```python
from build123d import *

# Parameters (mm, degrees)
F1_DEPTH = 7
F3_D     = 10


with BuildPart() as f1:
    # F0 (on Front) → F1 (new body)
    with BuildSketch(Plane.XZ):
        Polygon((7.5, -4.330127), (7.5, 4.330127), (0, 8.660254), (-7.5, 4.330127), (-7.5, -4.330127), (0, -8.660254), align=None)
    extrude(amount=F1_DEPTH)

    # F3 (through all)
    with Locations(Plane.XZ.offset(7)):
        with Locations((0, 0)):
            Hole(F3_D / 2)


solid = f1.part
```
The model under review builds one solid part; all positions refer to its coordinate system, in mm. Round coordinates to 2 decimals unless told otherwise and drop trailing zeros. Order: outer loops, then holes, each group sorted by start corner. A loop starts at its lowest first (then second) coordinate and runs counter-clockwise, first axis right, second up. Notation, with made-up numbers: (-28, 25.25) -> (23, 25.25) arc R15 ccw to (23, 50.25) -> close; hole circle Ø10 at (83.25, 73.5). An arc over 180 degrees is marked (long way). One line per item, written item: value. Start each with the question number.
Q1. Take a section at A-A (z = 0). Write out the cut boundary in (x, y), and give its area (3 significant figures).
Q2. Take a section at B-B (y = -3). Write out the cut boundary in (x, z).
Q3. Mouldability with a two-part tool opening along X and no side actions: class faces 1 (the face through (1.08, -3.45, -4.88)), 2 (the face through (-5, 0, -2)), 3 (the face through (-3.802, -3.451, -6.465)), 4 (the face through (7.5, -3, 0)) as released by +X, released by -X, zero draft, split by the parting line, or undercut.
Q4. Wall thickness on line 1 (Z direction, x = -4.25, y = -5.5); line 2 (X direction, y = -5, z = -4.5); line 3 (X direction, y = -0.75, z = -1.25): over which ranges is each line inside the solid? List them lowest first.
Q5. Clearance check with a flat-ended pin moving along its axis: pin 1 Ø1 at (x, y) = (2, -4.5) entering from +Z. State where the tip first meets the part, or that it passes through.
Q6. Take a section at D-D (z = 7.75). Write out the cut boundary in (x, y), and give its area (3 significant figures).
Q7. Take a section at C-C (x = -1.25). Write out the cut boundary in (y, z), and give its area (3 significant figures).
Reported:
1. outline: (-7.5, -7) -> (-5, -7) -> (-5, 0) -> (-7.5, 0) -> close; (5, -7) -> (7.5, -7) -> (7.5, 0) -> (5, 0) -> close
1. area: 35.0 mm2
2. outline: (-7.5, -4.33) -> (0, -8.66) -> (7.5, -4.33) -> (7.5, 4.33) -> (0, 8.66) -> (-7.5, 4.33) -> close; hole circle Ø10 at (0, 0)
3. face 1: undercut
3. face 2: zero draft
3. face 3: released by -X
3. face 4: released by +X
4. line 1: z = -6.21 to -2.63, 2.63 to 6.21
4. line 2: x = -7.21 to -2.18, 2.18 to 7.21
4. line 3: x = -7.5 to -4.84, 4.84 to 7.5
5. pin 1: stops at z = 7.79
6. outline: (-1.58, -7) -> (1.58, -7) -> (1.58, 0) -> (-1.58, 0) -> close
6. area: 22.1 mm2
7. outline: (-7, -7.94) -> (0, -7.94) -> (0, -4.84) -> (-7, -4.84) -> close; (-7, 4.84) -> (0, 4.84) -> (0, 7.94) -> (-7, 7.94) -> close
7. area: 43.4 mm2
